For this review, use the dimensioned drawing (mm, ordinates from the lowest corner) and the shaded views. A direction names the side the tool comes from. Round coordinates to 2 decimals unless told otherwise and drop trailing zeros. Order: outer loops, then holes, each group sorted by start corner. A loop starts at its lowest first (then second) coordinate and runs counter-clockwise, first axis right, second up. Notation, with made-up numbers: (84.25, 11) - (132.25, 11) arc R28 cw to (132.25, 40) - close; hole circle Ø8 at (-8.75, 81.25). An arc over 180 degrees is marked (long way). Write item = value, one per line.
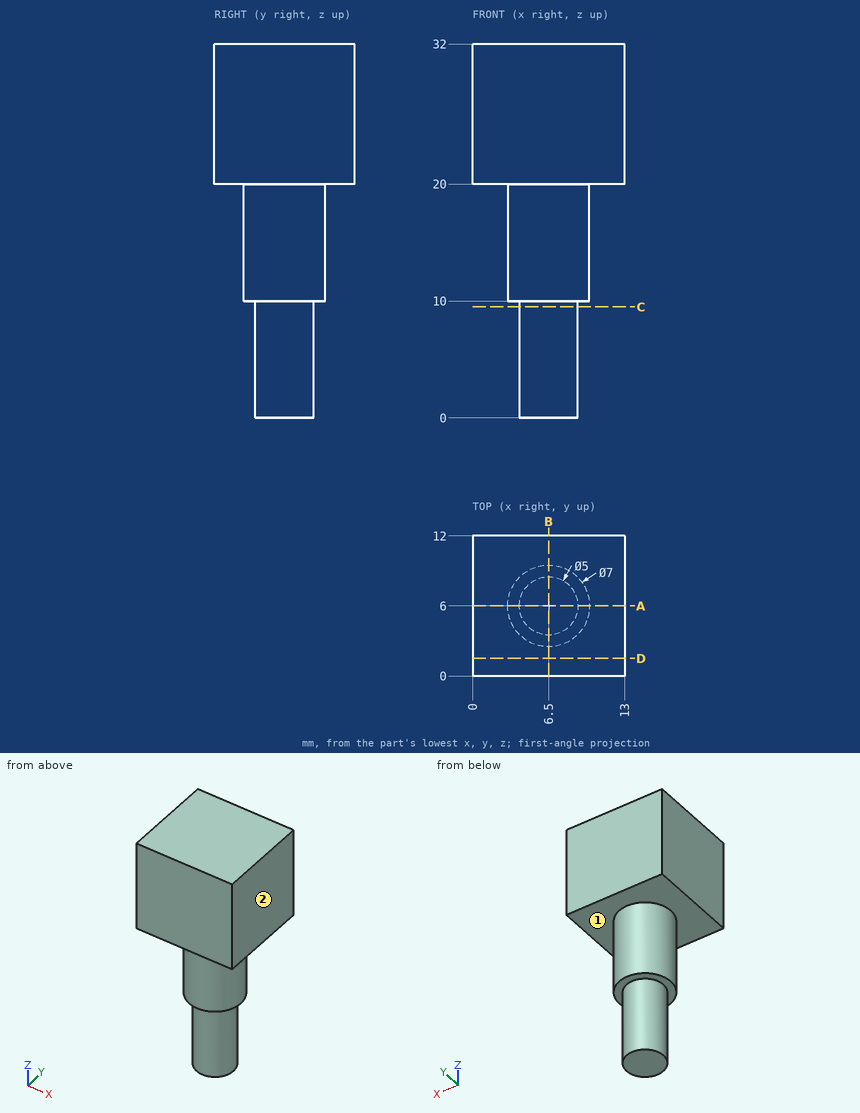
1) We need section A-A on y = 6. Write out the cut boundary in (x, z), and give its area (3 significant figures).
Findings:
outline = (0, 20) - (3, 20) - (3, 10) - (4, 10) - (4, 0) - (9, 0) - (9, 10) - (10, 10) - (10, 20) - (13, 20) - (13, 32) - (0, 32) - close
area = 276 mm^2
2) We need section D-D on y = 1.5. Write out the cut boundary in (x, z), and give its area (3 significant figures).
Findings:
outline = (0, 20) - (13, 20) - (13, 32) - (0, 32) - close
area = 156 mm^2
3) Clearance check with flat-ended pins moving along their axes: pin 1 Ø6 at (x, z) = (9.5, 7.5) entering from -Y; pin 2 Ø1 at (y, z) = (3.5, 5.5) entering from +X. State where each tip first meets the part, or that it passes through.
Findings:
pin_1 = 2.77
pin_2 = 8
4) To check wall thickness, follow L1, parallel to Z at x = 3.5, y = 6.75; L2, parallel to Z at x = 10, y = 4.75; L3, parallel to Y at x = 6.5, z = 17. State the ranges of each line that lie inside material, in increasing order. Write a range as from..to.
Findings:
L1 = 10..32
L2 = 20..32
L3 = 2.5..9.5
5) For the marked faces 1 and 2, list the 3-axis set-ups (+Z, -Z, +X, -X, +Y, -Y) from which the entire face can be reached by the end or side of a thin tool; tool diameter is ignored.
Findings:
face_1 = -Z
face_2 = +Z, -Z, +X, +Y, -Y
6) We need section B-B on x = 6.5. Write out the cut boundary in (y, z), and give its area (3 significant figures).
Findings:
outline = (0, 20) - (2.5, 20) - (2.5, 10) - (3.5, 10) - (3.5, 0) - (8.5, 0) - (8.5, 10) - (9.5, 10) - (9.5, 20) - (12, 20) - (12, 32) - (0, 32) - close
area = 264 mm^2
7) We need section C-C on z = 9.5. Write out the cut boundary in (x, y), and give its area (3 significant figures).
Findings:
outline = circle Ø5 at (6.5, 6)
area = 19.6 mm^2
